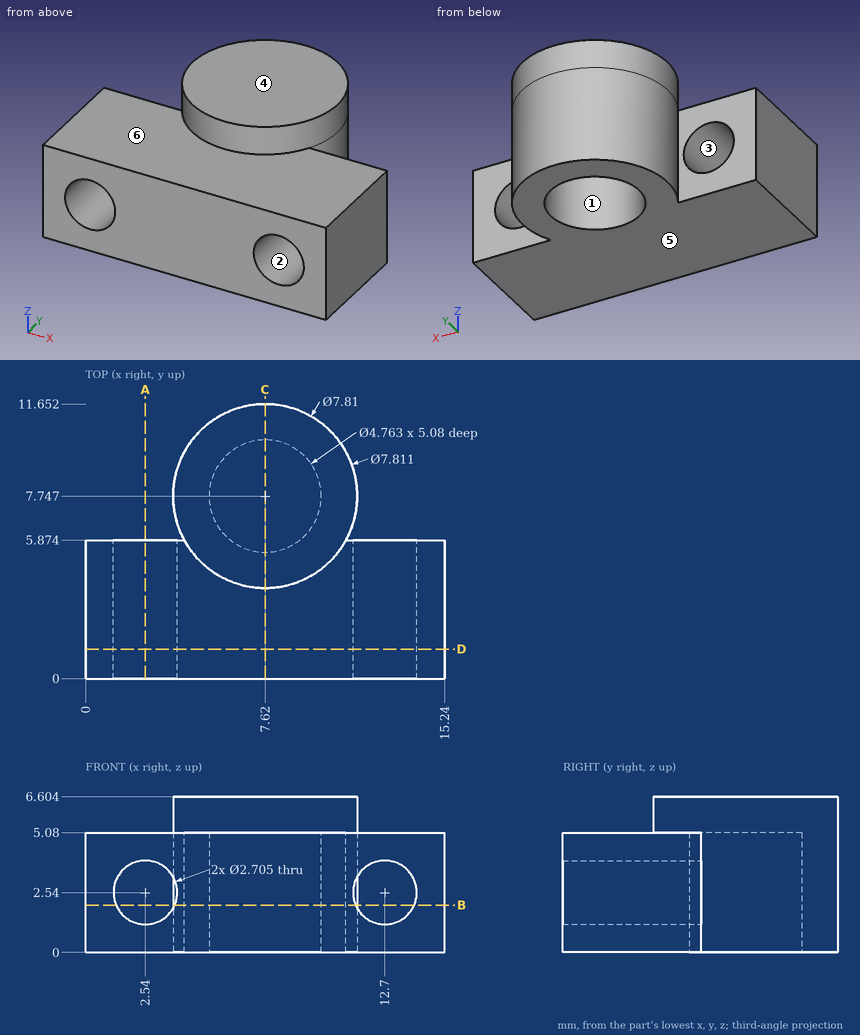
Verification items for this drawing (mm, ordinates from the low corner). A direction names the side the tool comes from. Round coordinates to 2 decimals unless told otherwise and drop trailing zeros. Write each loop counter-clockwise with the first axis right and the second up, starting at its lowest first coordinate (ties: lowest second). Pieces come first, ordered by that corner, then holes. Notation, with made-up numbers: (4, 15.25) - (28, 15.25) arc R24 cw to (28, 44.25) - close; hole circle Ø7 at (-21.5, 84). An arc over 180 degrees is marked (long way). Answer as a JSON object with one key per item and string values. Group by question number.
Q1. Tool access check on the marked faces 5 and 6. Record the directions out of +Z, -Z, +X, -X, +Y, -Y that give a thin tool (end or side, any length) a straight path to the whole face; none if there is none.
Q2. Mould release check, pull along Z, two halves, no side actions. Record for the marked faces 1, 2, 3 and 4: released by +Z, released by -Z, zero draft, split by the parting line, or undercut.
Q3. Section check C-C, the plane x = 7.62. Enter the section's corners in (y, z) (1 decimal).
Q4. Section check B-B, the plane z = 2. Enter the section's corners in (x, y) (1 decimal).
Q5. Section check D-D, the plane y = 1.25. Enter the section's corners in (x, z) (1 decimal).
Q6. Section check A-A, the plane x = 2.54. Enter the section's corners in (y, z).
Q7. Thickness scan on line 1 (Z direction, x = 12.7, y = 2.6); line 2 (Y direction, x = 7.62, z = 3.85) (1 decimal); line 3 (X direction, y = 1.7, z = 2.54). Record the ranges inside material, lowest first.
Q8. Go/stop test with flat-tipped pins: pin 1 Ø3.5 at (x, z) = (12.5, 2.5) entering from +Y; pin 2 Ø1.4 at (x, y) = (7, 8.5) entering from -Z; pin 3 Ø1.8 at (x, y) = (9.5, 2) entering from +Z. Record where each tip stops, or that it passes through.
Found:
{
 "1": {"face 5": "-Z, +X, -X, +Y, -Y", "face 6": "+Z, -Y"},
 "2": {"face 1": "zero draft", "face 2": "undercut", "face 3": "undercut", "face 4": "released by +Z"},
 "3": {"outline": "(0, 0) - (5.4, 0) - (5.4, 5.1) - (10.1, 5.1) - (10.1, 0) - (11.7, 0) - (11.7, 6.6) - (3.8, 6.6) - (3.8, 5.1) - (0, 5.1) - close"},
 "4": {"outline": "(0, 0) - (1.3, 0) - (1.3, 5.9) - (0, 5.9) - close; (3.8, 0) - (11.5, 0) - (11.5, 5.9) - (11, 5.9) arc R3.9 ccw (long way) to (4.2, 5.9) - (3.8, 5.9) - close; (13.9, 0) - (15.2, 0) - (15.2, 5.9) - (13.9, 5.9) - close; hole circle Ø4.8 at (7.6, 7.7)"},
 "5": {"outline": "(0, 0) - (15.2, 0) - (15.2, 5.1) - (0, 5.1) - close; hole circle Ø2.7 at (2.5, 2.5); hole circle Ø2.7 at (12.7, 2.5)"},
 "6": {"outline": "(0, 0) - (5.87, 0) - (5.87, 1.19) - (0, 1.19) - close; (0, 3.89) - (5.87, 3.89) - (5.87, 5.08) - (0, 5.08) - close"},
 "7": {"line 1": "z = 0 to 1.19, 3.89 to 5.08", "line 2": "y = 0 to 5.4, 10.1 to 11.7", "line 3": "x = 0 to 1.19, 3.89 to 11.35, 14.05 to 15.24"},
 "8": {"pin 1": "stops at y = 10.08", "pin 2": "stops at z = 5.08", "pin 3": "stops at z = 5.08"}
}
